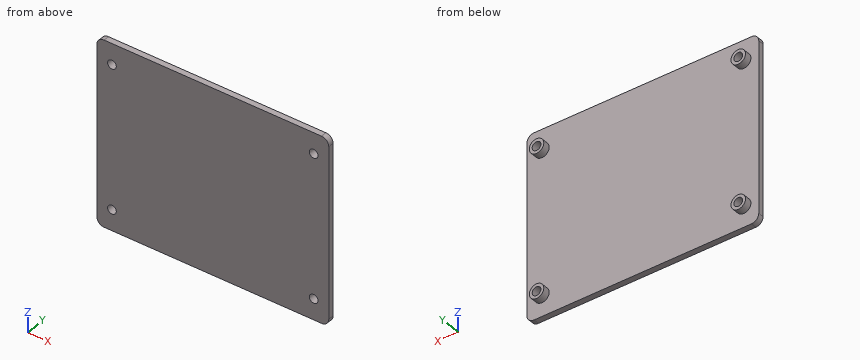
from build123d import *

# Parameters (mm, degrees)
SKETCH1_W           = 80
SKETCH1_H           = 64
BOSS_EXTRUDE1_DEPTH = 2
FILLET1_R           = 2.5
SKETCH2_R           = 1.5
CUT_EXTRUDE1_DEPTH  = 2
BOSS_EXTRUDE2_START = 2.5
SKETCH3_R           = 2.5
SKETCH3_R_2         = 1.5
BOSS_EXTRUDE2_DEPTH = 2.5


with BuildPart() as part:
    # Sketch1 → Boss-Extrude1 (new body)
    with BuildSketch(Plane(origin=(0, 0, 0), x_dir=(1, 0, 0), z_dir=(0, 1, 0))):
        Rectangle(SKETCH1_W, SKETCH1_H)
    extrude(amount=BOSS_EXTRUDE1_DEPTH)

    # Fillet1
    fillet1_edges = [part.edges().sort_by_distance(p)[0] for p in [
        (40, 1, 32),
        (-40, 1, 32),
        (-40, 1, -32),
        (40, 1, -32),
    ]]
    fillet(fillet1_edges, radius=FILLET1_R)

    # Sketch2 → Cut-Extrude1 (cut)
    with BuildSketch(Plane(origin=(-9.018883196, 2, 9.463275917), x_dir=(1, 0, 0), z_dir=(0, 1, 0))):
        with Locations(Location((-25.781116804, 34.263275917, 0), (0, 0, 270))):
            Circle(SKETCH2_R)
        with Locations(Location((43.818883196, 34.263275917, 0), (0, 0, 270))):
            Circle(SKETCH2_R)
        with Locations(Location((43.818883196, -15.336724083, 0), (0, 0, 270))):
            Circle(SKETCH2_R)
        with Locations(Location((-25.781116804, -15.336724083, 0), (0, 0, 270))):
            Circle(SKETCH2_R)
    extrude(amount=-CUT_EXTRUDE1_DEPTH, mode=Mode.SUBTRACT)

    # Sketch3 → Boss-Extrude2 (add)
    # profile 1 of 4: a face of its own
    with BuildSketch(Plane(origin=(0, 2, 0), x_dir=(1, 0, 0), z_dir=(0, 1, 0)).offset(BOSS_EXTRUDE2_START)):
        with Locations(Location((-34.8, 24.8, 0), (0, 0, 90))):
            Circle(SKETCH3_R)
        with Locations(Location((-34.8, 24.8, 0), (0, 0, 270))):
            Circle(SKETCH3_R_2, mode=Mode.SUBTRACT)
    # profile 2 of 4: a face of its own
    with BuildSketch(Plane(origin=(0, 2, 0), x_dir=(1, 0, 0), z_dir=(0, 1, 0)).offset(BOSS_EXTRUDE2_START)):
        with Locations(Location((-34.8, -24.8, 0), (0, 0, 90))):
            Circle(SKETCH3_R)
        with Locations(Location((-34.8, -24.8, 0), (0, 0, 270))):
            Circle(SKETCH3_R_2, mode=Mode.SUBTRACT)
    # profile 3 of 4: a face of its own
    with BuildSketch(Plane(origin=(0, 2, 0), x_dir=(1, 0, 0), z_dir=(0, 1, 0)).offset(BOSS_EXTRUDE2_START)):
        with Locations(Location((34.8, 24.8, 0), (0, 0, 90))):
            Circle(SKETCH3_R)
        with Locations(Location((34.8, 24.8, 0), (0, 0, 270))):
            Circle(SKETCH3_R_2, mode=Mode.SUBTRACT)
    # profile 4 of 4: a face of its own
    with BuildSketch(Plane(origin=(0, 2, 0), x_dir=(1, 0, 0), z_dir=(0, 1, 0)).offset(BOSS_EXTRUDE2_START)):
        with Locations(Location((34.8, -24.8, 0), (0, 0, 90))):
            Circle(SKETCH3_R)
        with Locations(Location((34.8, -24.8, 0), (0, 0, 270))):
            Circle(SKETCH3_R_2, mode=Mode.SUBTRACT)
    extrude(amount=-BOSS_EXTRUDE2_DEPTH)


solid = part.part
Source: CAD feature listing. Evaluate the final solid. Frame: model axes, mm. Coordinates: 2 decimals unless noted, no trailing zeros. Write each loop counter-clockwise with the first axis right and the second up, starting at its lowest first coordinate (ties: lowest second). Pieces come first, ordered by that corner, then holes. Notation, with made-up numbers: M 59,23 L 113,23 A20 cw 113,49 Z; hole C -19.75,37.5 d5. An arc over 180 degrees is marked long. Use a Markdown table: item, result.
1) Section B-B, the plane y = 3.15. Output: boundary loops of the cut face in (x, z), then the cut area to 3 significant figures.
Conclusion:
| item | result |
|---|---|
| outline | C -34.8,-24.8 d5; C -34.8,24.8 d5; C 34.8,-24.8 d5; C 34.8,24.8 d5; hole C -34.8,-24.8 d3; hole C -34.8,24.8 d3; hole C 34.8,-24.8 d3; hole C 34.8,24.8 d3 |
| area | 50.3 mm^2 |
2) Section D-D, the plane x = -5. Output: boundary loops of the cut face in (y, z), then the cut area to 3 significant figures.
Conclusion:
| item | result |
|---|---|
| outline | M 0,-32 L 2,-32 L 2,32 L 0,32 Z |
| area | 128 mm^2 |
3) First-contact query: pin 1 Ø4 at (x, z) = (-2.5, 15) entering from +Y. Flat tip, straight axial feed; report the tip coordinate or a pass-through.
Conclusion:
| item | result |
|---|---|
| pin 1 | stops at y = 2 |
4) Ray query, L1, parallel to X at y = 3.5, z = 24.8; L2, parallel to X at y = 1.4, z = -24.8; L3, parallel to Z at x = 35, y = 2.25. Return the intervals inside material, ascending.
Conclusion:
| item | result |
|---|---|
| L1 | x = -37.3 to -36.3, -33.3 to -32.3, 32.3 to 33.3, 36.3 to 37.3 |
| L2 | x = -40 to -36.3, -33.3 to 33.3, 36.3 to 40 |
| L3 | z = -27.29 to -26.29, -23.31 to -22.31, 22.31 to 23.31, 26.29 to 27.29 |
5) Section C-C, the plane z = 24.8. Output: boundary loops of the cut face in (x, y), then the cut area to 3 significant figures.
Conclusion:
| item | result |
|---|---|
| outline | M -40,0 L -36.3,0 L -36.3,4.5 L -37.3,4.5 L -37.3,2 L -40,2 Z; M -33.3,0 L 33.3,0 L 33.3,4.5 L 32.3,4.5 L 32.3,2 L -32.3,2 L -32.3,4.5 L -33.3,4.5 Z; M 36.3,0 L 40,0 L 40,2 L 37.3,2 L 37.3,4.5 L 36.3,4.5 Z |
| area | 158 mm^2 |
6) Section A-A, the plane x = 34.8. Output: boundary loops of the cut face in (y, z).
Conclusion:
| item | result |
|---|---|
| outline | M 0,-32 L 2,-32 L 2,-27.3 L 4.5,-27.3 L 4.5,-26.3 L 0,-26.3 Z; M 0,-23.3 L 4.5,-23.3 L 4.5,-22.3 L 2,-22.3 L 2,22.3 L 4.5,22.3 L 4.5,23.3 L 0,23.3 Z; M 0,26.3 L 4.5,26.3 L 4.5,27.3 L 2,27.3 L 2,32 L 0,32 Z |
